Input: part model. Units: mm. Frame: model coordinates. A direction names the side the tool comes from. Round coordinates to 2 decimals unless told otherwise and drop trailing zeros. Loops run counter-clockwise (first coordinate to the right, second up) from the corner with the lowest first, then second, coordinate; pieces in that order, holes last. Notation, with made-up numbers: (-39.75, -14) -> (-18.75, -14) arc R15 cw to (-18.75, -9) -> close; hole circle Ø1 at (54, -26). An arc over 180 degrees is marked (long way). One line per question, with ' | ' between items. Start each with the question number.
Q1. Access query for faces 1 (the face through (-17.299, -2, -14)), 2 (the face through (9, 1, 7.92)), 3 (the face through (9.701, -2, 20)), 4 (the face through (-19.549, 1, 3)), 5 (the face through (-3, -4.6, -14)). Directions: +Z, -Z, +X, -X, +Y, -Y. A direction counts if a zero-diameter tool reaches every point of the face in a straight line with its end or side. Return the directions, or none.
Q2. Material intervals for L1, parallel to Z at x = -5, y = -2.75; L2, parallel to Z at x = 5, y = -4; L3, parallel to Y at x = 9, z = 11.5, sorted ascending.
Q3. Cut plane A-A on z = 0.5. Return loops of the section in (x, y).
Q4. Cut plane D-D on z = 14. Return loops of the section in (x, y).
Q5. Cut plane B-B on y = -2. Return loops of the section in (x, z).
Q6. Mould query, pull axis X, two halves, no side actions, for faces 6 (the face through (11, -2, 21.2)), 7 (the face through (-9.299, -2, 20)), 8 (the face through (4.701, -2, 20)). Classes: pulls with the +X half, pulls with the -X half, needs draft (parallel to the pull), parting line crosses it, or undercut.
Q7. Contact query for flat-ended pins moving along their axis: P1, Ø1.8, axis at x = -2, y = -3.5, coming from the -Z side; P2, Ø2, axis at x = -7, y = -2.5, coming from the +Z side; P3, Ø2, axis at y = -3, z = -13, coming from the +X side. Output: stop coordinate, or through.
Q8. Cut plane C-C on x = -1. Return loops of the section in (y, z), and give its area (3 significant figures).
from build123d import *

# Parameters (mm, degrees)
SKETCH1_W           = 34.5
SKETCH1_H           = 40.5
BOSS_EXTRUDE1_DEPTH = 1.7
SKETCH2_W           = 3.66
SKETCH2_H           = 9.44
CUT_EXTRUDE1_DEPTH  = 1.7
FILLET1_R           = 1
FILLET2_R           = 1
FILLET3_R           = 1
FILLET4_R           = 1
FILLET5_R           = 1
FILLET6_R           = 1
FILLET7_R           = 1
FILLET8_R           = 1
SKETCH3_W           = 30
SKETCH3_H           = 1.6
BOSS_EXTRUDE2_DEPTH = 4.6
SKETCH4_W           = 3
SKETCH4_H           = 1.7
SKETCH4_W_2         = 14
BOSS_EXTRUDE3_DEPTH = 4.6
BOSS_EXTRUDE4_START = -14.75
BOSS_EXTRUDE4_DEPTH = 5
FILLET9_R           = 1
FILLET10_R          = 1
FILLET11_R          = 1


with BuildPart() as part:
    # Sketch1 → Boss-Extrude1 (new body)
    with BuildSketch(Plane(origin=(0, 0, 0), x_dir=(1, 0, 0), z_dir=(0, 1, 0))):
        with Locations((-2.298701299, -3.199675325)):
            Rectangle(SKETCH1_W, SKETCH1_H)
    extrude(amount=BOSS_EXTRUDE1_DEPTH)

    # Sketch2 → Cut-Extrude1 (cut)
    with BuildSketch(Plane(origin=(0, 1.7, 0), x_dir=(1, 0, 0), z_dir=(0, 1, 0))):
        with Locations((8.851298701, -3.199675325)):
            Rectangle(SKETCH2_W, SKETCH2_H)
    extrude(amount=-CUT_EXTRUDE1_DEPTH, mode=Mode.SUBTRACT)

    # Fillet1
    fillet1_edges = [part.edges().sort_by_distance(p)[0] for p in [
        (14.951298701, 0.85, 23.449675325),
    ]]
    fillet(fillet1_edges, radius=FILLET1_R)

    # Fillet2
    fillet2_edges = [part.edges().sort_by_distance(p)[0] for p in [
        (14.951298701, 0.85, -17.050324675),
    ]]
    fillet(fillet2_edges, radius=FILLET2_R)

    # Fillet3
    fillet3_edges = [part.edges().sort_by_distance(p)[0] for p in [
        (-19.548701299, 0.85, -17.050324675),
    ]]
    fillet(fillet3_edges, radius=FILLET3_R)

    # Fillet4
    fillet4_edges = [part.edges().sort_by_distance(p)[0] for p in [
        (-19.548701299, 0.85, 23.449675325),
    ]]
    fillet(fillet4_edges, radius=FILLET4_R)

    # Fillet5
    fillet5_edges = [part.edges().sort_by_distance(p)[0] for p in [
        (7.021298701, 0.85, 7.919675325),
    ]]
    fillet(fillet5_edges, radius=FILLET5_R)

    # Fillet6
    fillet6_edges = [part.edges().sort_by_distance(p)[0] for p in [
        (7.021298701, 0.85, -1.520324675),
    ]]
    fillet(fillet6_edges, radius=FILLET6_R)

    # Fillet7
    fillet7_edges = [part.edges().sort_by_distance(p)[0] for p in [
        (10.681298701, 0.85, 7.919675325),
    ]]
    fillet(fillet7_edges, radius=FILLET7_R)

    # Fillet8
    fillet8_edges = [part.edges().sort_by_distance(p)[0] for p in [
        (10.681298701, 0.85, -1.520324675),
    ]]
    fillet(fillet8_edges, radius=FILLET8_R)

    # Sketch3 → Boss-Extrude2 (add)
    with BuildSketch(Plane.XZ):
        with Locations((-2.298701299, -14.000324675)):
            Rectangle(SKETCH3_W, SKETCH3_H)
    extrude(amount=BOSS_EXTRUDE2_DEPTH)

    # Sketch4 → Boss-Extrude3 (add)
    with BuildSketch(Plane.XZ):
        with Locations((11.201298701, 20.349675325)):
            Rectangle(SKETCH4_W, SKETCH4_H)
        with Locations((-2.298701299, 20.349675325)):
            Rectangle(SKETCH4_W_2, SKETCH4_H)
    extrude(amount=BOSS_EXTRUDE3_DEPTH)

    # Sketch5 → Boss-Extrude4 (add)
    with BuildSketch(Plane(origin=(14.951298701, 0, 0), x_dir=(0, 0, -1), z_dir=(1, 0, 0)).offset(BOSS_EXTRUDE4_START)):
        Polygon((14.800324675, -2.5), (14.800324675, -4), (15.550324675, -2.75), (15.550324675, -2.5), align=None)
        Polygon((-21.949675325, -2.5), (-21.199675325, -2.5), (-21.199675325, -4), (-21.949675325, -2.75), align=None)
    extrude(amount=-BOSS_EXTRUDE4_DEPTH)

    # Fillet9
    fillet9_edges = [part.edges().sort_by_distance(p)[0] for p in [
        (11.201298701, 0, 19.499675325),
    ]]
    fillet(fillet9_edges, radius=FILLET9_R)

    # Fillet10
    fillet10_edges = [part.edges().sort_by_distance(p)[0] for p in [
        (-2.298701299, 0, 19.499675325),
    ]]
    fillet(fillet10_edges, radius=FILLET10_R)

    # Fillet11
    fillet11_edges = [part.edges().sort_by_distance(p)[0] for p in [
        (-2.298701299, 0, -13.200324675),
    ]]
    fillet(fillet11_edges, radius=FILLET11_R)


solid = part.part
Results:
1) face 1: +Z, -Z, -X, -Y | face 2: +Y, -Y | face 3: +Z, -Y | face 4: +Z, -Z, -X, +Y, -Y | face 5: +Z, -Z, +X, -X, -Y
2) L1: -14.8 to -13.2, 19.5 to 21.2 | L2: -14.8 to -13.2 | L3: 0 to 1.7
3) outline: (-19.55, 0) -> (7.02, 0) -> (7.02, 1.7) -> (-19.55, 1.7) -> close; (10.68, 0) -> (14.95, 0) -> (14.95, 1.7) -> (10.68, 1.7) -> close
4) outline: (-19.55, 0) -> (14.95, 0) -> (14.95, 1.7) -> (-19.55, 1.7) -> close
5) outline: (-17.3, -14.8) -> (12.7, -14.8) -> (12.7, -13.2) -> (-17.3, -13.2) -> close; (-9.3, 19.5) -> (4.7, 19.5) -> (4.7, 21.2) -> (-9.3, 21.2) -> close; (9.7, 19.5) -> (12.7, 19.5) -> (12.7, 21.2) -> (9.7, 21.2) -> close
6) face 6: needs draft | face 7: pulls with the -X half | face 8: undercut
7) P1: z = -15.55 | P2: z = 21.2 | P3: x = 12.7
8) outline: (-4.6, -14.8) -> (-4, -14.8) -> (-2.75, -15.55) -> (-2.5, -15.55) -> (-2.5, -14.8) -> (0, -14.8) -> (0, -17.05) -> (1.7, -17.05) -> (1.7, 23.45) -> (0, 23.45) -> (0, 21.2) -> (-2.5, 21.2) -> (-2.5, 21.95) -> (-2.75, 21.95) -> (-4, 21.2) -> (-4.6, 21.2) -> (-4.6, 19.5) -> (-1, 19.5) arc R1 cw to (0, 18.5) -> (0, -12.2) arc R1 cw to (-1, -13.2) -> (-4.6, -13.2) -> close | area: 85.8 mm^2
